```python
from build123d import *

# Parameters (mm, degrees)
PAD_DEPTH          = 5
POLARPATTERN_COUNT = 4


with BuildPart() as part:
    # Sketch → Pad (new body, symmetric)
    with BuildSketch(Plane.XY):
        with BuildLine():
            Line((-4.9, 10), (-3.1, 8.2))
            Line((-3.1, 8.2), (-5.49934, 8.2))
            Line((-5.49934, 8.2), (-5.49934, 6.56))
            Line((-5.49934, 6.56), (-2.84, 3.90066))
            Line((-2.84, 3.90066), (0, 3.90066))
            Line((0, 3.90066), (0, 2.1))
            ThreePointArc((0, 2.1), (-1.484924, 1.484924), (-2.1, 0))
            Line((-3.90066, 0), (-2.1, 0))
            Line((-3.90066, 0), (-3.90066, 2.84))
            Line((-3.90066, 2.84), (-6.56, 5.49934))
            Line((-6.56, 5.49934), (-8.2, 5.49934))
            Line((-8.2, 5.49934), (-8.2, 3.1))
            Line((-8.2, 3.1), (-10, 4.9))
            Line((-10, 4.9), (-10, 9))
            ThreePointArc((-9, 10), (-9.707107, 9.707107), (-10, 9))
            Line((-4.9, 10), (-9, 10))
        make_face()
    pad = extrude(amount=PAD_DEPTH, both=True)

    # PolarPattern: Pad ×4 about axis
    polarpattern_axis = Axis((0, 0, 0), (0, 0, 1))
    for i in range(1, POLARPATTERN_COUNT):
        add(pad.rotate(polarpattern_axis, i * 360 / POLARPATTERN_COUNT))


solid = part.part
```
Geometry check sheet. Reference: the model listing, model coordinates, mm. A direction names the side the tool comes from. Coordinates: 2 decimals unless noted, no trailing zeros. Order: outer loops, then holes, each group sorted by start corner. A loop starts at its lowest first (then second) coordinate and runs counter-clockwise, first axis right, second up.
Item 1: Scan lines: line 1 along X through (y, z) = (-7.75, -1.25); line 2 along X through (y, z) = (-5, 4.25); line 3 along Y through (x, z) = (-2.5, 1). Record each from-to range of solid material in increasing order.
Item 2: Section check A-A (y = -0.5). Enter the section's corners in (x, z).
Item 3: Tool access check on faces 4 (the flat face through (-9.1, 4, 0.1)), 5 (the flat face through (-4, 9.1, 0.1)), 6 (the flat face through (-4.19, 5.25, 0.07)). Record the directions out of +Z, -Z, +X, -X, +Y, -Y that give a thin tool (end or side, any length) a straight path to the whole face; none if there is none.
Item 4: Depth check by flat-ended pin: pin 1 (2 mm diameter, centred on x = -5, y = -1.5, fed in from -Z); pin 2 (6 mm diameter, centred on y = 1, z = 0, fed in from -X); pin 3 (0.7 mm diameter, centred on x = -4, z = -0.5, fed in from -Y); pin 4 (6 mm diameter, centred on y = 1, z = 2.5, fed in from +X). Enter the tip coordinate at first touch or a pass-through.
Item 5: Section check C-C (y = 5.25). Enter the section's corners in (x, z).
Item 6: Section check B-B (x = 1). Enter the section's corners in (y, z).
Item 7: Mould release check, pull along Y, two halves, no side actions. Record for faces 1 (the flat face through (7, 10, 0)), 2 (the flat face through (-5.21, 4.15, 0.07)), 3 (the flat face through (2.4, -0.1, 5)): released by +Y, released by -Y, zero draft, split by the parting line, or undercut.
Check sheet entries:
1. line 1: x = -10 to -5.5, 5.5 to 10
1. line 2: x = -10 to -8.2, -6.06 to -3.94, 3.94 to 6.06, 8.2 to 10
1. line 3: y = -3.9 to 3.9
2. outline: (-3.9, -5) - (-2.04, -5) - (-2.04, 5) - (-3.9, 5) - close; (2.04, -5) - (3.9, -5) - (3.9, 5) - (2.04, 5) - close
3. face 4: +Z, -Z, -X
3. face 5: +Z, -Z, +Y
3. face 6: +Z, -Z
4. pin 1: passes through
4. pin 2: stops at x = -9.1
4. pin 3: stops at y = -9.45
4. pin 4: stops at x = 9.1
5. outline: (-10, -5) - (-8.2, -5) - (-8.2, 5) - (-10, 5) - close; (-6.31, -5) - (-4.19, -5) - (-4.19, 5) - (-6.31, 5) - close; (4.19, -5) - (6.31, -5) - (6.31, 5) - (4.19, 5) - close; (8.2, -5) - (10, -5) - (10, 5) - (8.2, 5) - close
6. outline: (-3.9, -5) - (-1.85, -5) - (-1.85, 5) - (-3.9, 5) - close; (1.85, -5) - (3.9, -5) - (3.9, 5) - (1.85, 5) - close
7. face 1: released by +Y
7. face 2: undercut
7. face 3: zero draft
